from build123d import *

# Parameters (mm, degrees)
SKETCH1_R           = 5
BOSS_EXTRUDE1_DEPTH = 2
SKETCH2_R           = 7
BOSS_EXTRUDE2_DEPTH = 7
SKETCH3_R           = 3
BOSS_EXTRUDE3_DEPTH = 1.5
SKETCH4_R           = 1
BOSS_EXTRUDE4_DEPTH = 8
SKETCH5_R           = 0.4
CUT_EXTRUDE1_DEPTH  = 8
SKETCH7_R           = 0.35
CUT_EXTRUDE2_DEPTH  = 0.4


with BuildPart() as part:
    # Sketch1 → Boss-Extrude1 (new body)
    with BuildSketch(Plane.XY):
        Circle(SKETCH1_R)
    extrude(amount=BOSS_EXTRUDE1_DEPTH)

    # Sketch2 → Boss-Extrude2 (add)
    with BuildSketch(Plane.XY.offset(2)):
        Circle(SKETCH2_R)
    extrude(amount=BOSS_EXTRUDE2_DEPTH)

    # Sketch3 → Boss-Extrude3 (add)
    with BuildSketch(Plane.XY.offset(9)):
        Circle(SKETCH3_R)
    extrude(amount=BOSS_EXTRUDE3_DEPTH)

    # Sketch4 → Boss-Extrude4 (add)
    with BuildSketch(Plane(origin=(6, 0, 0), x_dir=(0, 0, -1), z_dir=(1, 0, 0))):
        with Locations((-3.75, 0)):
            Circle(SKETCH4_R)
    extrude(amount=BOSS_EXTRUDE4_DEPTH)

    # Sketch5 → Cut-Extrude1 (cut)
    with BuildSketch(Plane(origin=(14, 0, 0), x_dir=(0, 0, -1), z_dir=(1, 0, 0))):
        with Locations((-3.75, 0)):
            Circle(SKETCH5_R)
    extrude(amount=-CUT_EXTRUDE1_DEPTH, mode=Mode.SUBTRACT)

    # Sketch7 → Cut-Extrude2 (cut)
    with BuildSketch(Plane(origin=(0, 0, 0), x_dir=(-1, 0, 0), z_dir=(0, 0, -1))):
        Circle(SKETCH7_R)
        with Locations((0, 2)):
            Circle(SKETCH7_R)
        with Locations((0, -2)):
            Circle(SKETCH7_R)
        with Locations((2, 0)):
            Circle(SKETCH7_R)
        with Locations((2, 2)):
            Circle(SKETCH7_R)
        with Locations((2, -2)):
            Circle(SKETCH7_R)
        with Locations((-2, 0)):
            Circle(SKETCH7_R)
        with Locations((-2, 2)):
            Circle(SKETCH7_R)
        with Locations((-2, -2)):
            Circle(SKETCH7_R)
    extrude(amount=-CUT_EXTRUDE2_DEPTH, mode=Mode.SUBTRACT)


solid = part.part
The listing builds one solid part. Answer for the finished solid, in the listing's coordinates (mm). A direction names the side the tool comes from. Give positions to 0.01 mm unless a question says otherwise; leave off trailing zeros. Write each loop counter-clockwise with the first axis right and the second up, starting at its lowest first coordinate (ties: lowest second). Pieces come first, ordered by that corner, then holes.
Item 1: Which of the six approach directions +Z, -Z, +X, -X, +Y, -Y give full straight-line access (tool end or side, diameter ignored) to faces 1 (the flat face through (1, -3, 9)), 2 (the flat face through (-2, 5, 2)), 3 (the cylindrical face through (10.41, 0.04, 4.75)), 4 (the flat face through (0, 0, 10.5))?
Item 2: Section A-A, the plane x = 0 is taken. Write down the section's boundary in (y, z).
Item 3: Flat-ended cylindrical pins translate along their axes: P1, Ø5, axis at x = -3, z = 5, coming from the -Y side; P2, Ø0.6, axis at x = -2, y = 0, coming from the -Z side; P3, Ø2, axis at y = 4, z = 8, coming from the +X side. Find the tip coordinate at first contact, or state that the pin passes through.
Item 4: Section D-D, the plane x = 12 is taken. Write down the section's boundary in (y, z), plus the area to 3 significant figures.
Item 5: Find the intervals of material crossed by line 1 along Y through (x, z) = (0, 0.2); line 2 along Y through (x, z) = (-2, 0.2); line 3 along Z through (x, y) = (-2, 4), in increasing order.
Item 6: Section C-C, the plane y = -2 is taken. Write down the section's boundary in (x, z), plus the area to 3 significant figures.
Item 7: Section B-B, the plane z = 3.75 is taken. Write down the section's boundary in (x, y).
Completed:
1. face 1: +Z
1. face 2: -Z
1. face 3: +X
1. face 4: +Z, +X, -X, +Y, -Y
2. outline: (-7, 2) - (-5, 2) - (-5, 0) - (-2.35, 0) - (-2.35, 0.4) - (-1.65, 0.4) - (-1.65, 0) - (-0.35, 0) - (-0.35, 0.4) - (0.35, 0.4) - (0.35, 0) - (1.65, 0) - (1.65, 0.4) - (2.35, 0.4) - (2.35, 0) - (5, 0) - (5, 2) - (7, 2) - (7, 9) - (3, 9) - (3, 10.5) - (-3, 10.5) - (-3, 9) - (-7, 9) - close
3. P1: stops at y = -6.98
3. P2: stops at z = 0.4
3. P3: stops at x = 6.32
4. outline: circle Ø2 at (0, 3.75); hole circle Ø0.8 at (0, 3.75)
4. area: 2.64 mm2
5. line 1: y = -5 to -2.35, -1.65 to -0.35, 0.35 to 1.65, 2.35 to 5
5. line 2: y = -4.58 to -2.35, -1.65 to -0.35, 0.35 to 1.65, 2.35 to 4.58
5. line 3: z = 0 to 9
6. outline: (-6.71, 2) - (-4.58, 2) - (-4.58, 0) - (-2.35, 0) - (-2.35, 0.4) - (-1.65, 0.4) - (-1.65, 0) - (-0.35, 0) - (-0.35, 0.4) - (0.35, 0.4) - (0.35, 0) - (1.65, 0) - (1.65, 0.4) - (2.35, 0.4) - (2.35, 0) - (4.58, 0) - (4.58, 2) - (6.71, 2) - (6.71, 9) - (2.24, 9) - (2.24, 10.5) - (-2.24, 10.5) - (-2.24, 9) - (-6.71, 9) - close
6. area: 118 mm2
7. outline: (6, -0.4) - (6, 0.4) - (14, 0.4) - (14, 1) - (6.93, 1) arc R7 ccw (long way) to (6.93, -1) - (14, -1) - (14, -0.4) - close
